For this review, take the finished solid that the model builds, in its own axes (mm). A direction names the side the tool comes from. Round coordinates to 2 decimals unless told otherwise and drop trailing zeros. Write each loop counter-clockwise with the first axis right and the second up, starting at its lowest first coordinate (ties: lowest second). Pieces come first, ordered by that corner, then holes. Notation, with made-up numbers: (63, 22.25) -> (77, 22.25) arc R17 cw to (77, 29.25) -> close; hole circle Ø10 at (83, -32). An arc over 180 degrees is marked (long way). Answer in a Markdown table with one row per item.
from build123d import *

# Parameters (mm, degrees)
SKETCH2_R           = 12.7
BOSS_EXTRUDE1_DEPTH = 38.1
CUT_EXTRUDE1_DEPTH  = 99.465595781


with BuildPart() as part:
    # Sketch2 → Boss-Extrude1 (new body)
    with BuildSketch(Plane.XY):
        with BuildLine():
            Line((-69.85, -36.5125), (69.85, -36.5125))
            Line((69.85, -36.5125), (69.85, -21.43125))
            Line((69.85, -21.43125), (29.639590069, -21.43125))
            ThreePointArc((29.639590069, -21.43125), (0, 36.576), (-29.639590069, -21.43125))
            Line((-29.639590069, -21.43125), (-69.85, -21.43125))
            Line((-69.85, -21.43125), (-69.85, -36.5125))
        make_face()
        with Locations(Location((0, 0, 0), (0, 0, 180))):
            Circle(SKETCH2_R, mode=Mode.SUBTRACT)
    extrude(amount=BOSS_EXTRUDE1_DEPTH)

    # Sketch3 → Cut-Extrude1 (cut, through all)
    with BuildSketch(Plane(origin=(0, -21.43125, 0), x_dir=(1, 0, 0), z_dir=(0, 1, 0))):
        with BuildLine():
            Line((-58.7375, -15.875), (-46.0375, -15.875))
            ThreePointArc((-46.0375, -15.875), (-42.8625, -19.05), (-46.0375, -22.225))
            Line((-46.0375, -22.225), (-58.7375, -22.225))
            ThreePointArc((-58.7375, -22.225), (-61.9125, -19.05), (-58.7375, -15.875))
        make_face()
    cut_extrude1 = extrude(amount=-CUT_EXTRUDE1_DEPTH, mode=Mode.SUBTRACT)

    # Mirror1: Cut-Extrude1 across plane
    add(cut_extrude1.mirror(Plane(origin=(0, 0, 0), x_dir=(0, 0, 1), z_dir=(1, 0, 0))), mode=Mode.SUBTRACT)


solid = part.part
1) For line 1 (Y direction, x = 0, z = 8.5); line 2 (Y direction, x = 57, z = 10.5); line 3 (Y direction, x = -33, z = 13), list the stretches that pass through material, from the lowest coordinate up. Write a range as [from, to].
Solved:
| item | result |
|---|---|
| line 1 | [-36.51, -12.7], [12.7, 36.58] |
| line 2 | [-36.51, -21.43] |
| line 3 | [-36.51, -21.43], [-15.77, 15.77] |
2) Consider section A-A on z = 19.05. State the section outline as (x, y) points.
Solved:
| item | result |
|---|---|
| outline | (-69.85, -36.51) -> (-61.91, -36.51) -> (-61.91, -21.43) -> (-69.85, -21.43) -> close; (-42.86, -36.51) -> (42.86, -36.51) -> (42.86, -21.43) -> (29.64, -21.43) arc R36.58 ccw (long way) to (-29.64, -21.43) -> (-42.86, -21.43) -> close; (61.91, -36.51) -> (69.85, -36.51) -> (69.85, -21.43) -> (61.91, -21.43) -> close; hole circle Ø25.4 at (0, 0) |
3) For faces 1 (the cylindrical face through (-5.86, 11.267, 18.783)), 2 (the cylindrical face through (-61.91, -28.87, 19.12)), list the 3-axis set-ups (+Z, -Z, +X, -X, +Y, -Y) from which the entire face can be reached by the end or side of a thin tool; tool diameter is ignored.
Solved:
| item | result |
|---|---|
| face 1 | +Z, -Z |
| face 2 | +Y, -Y |
4) Consider section D-D on y = 0. State the section outline as (x, z) points.
Solved:
| item | result |
|---|---|
| outline | (-36.58, 0) -> (-12.7, 0) -> (-12.7, 38.1) -> (-36.58, 38.1) -> close; (12.7, 0) -> (36.58, 0) -> (36.58, 38.1) -> (12.7, 38.1) -> close |
5) Consider section B-B on x = -53. State the section outline as (y, z) points (1 decimal).
Solved:
| item | result |
|---|---|
| outline | (-36.5, 0) -> (-21.4, 0) -> (-21.4, 15.9) -> (-36.5, 15.9) -> close; (-36.5, 22.2) -> (-21.4, 22.2) -> (-21.4, 38.1) -> (-36.5, 38.1) -> close |
6) Consider section C-C on y = -31.5. State how many separate pieces and enclosed holes the cut face has, then the cut area to 3 significant figures.
Solved:
| item | result |
|---|---|
| separate pieces | 1 |
| enclosed holes | 2 |
| area | 5,100 mm² |
7) Clearance check with flat-ended pins moving along their axes: pin 1 Ø6.5 at (x, y) = (-54.5, -32) entering from -Z; pin 2 Ø1 at (y, z) = (10.5, 26.5) entering from -X; pin 3 Ø3 at (y, z) = (9.5, 23) entering from -X; pin 4 Ø12 at (y, z) = (4, 26.5) entering from -X. State where each tip first meets the part, or that it passes through.
Solved:
| item | result |
|---|---|
| pin 1 | z = 0 |
| pin 2 | x = -35.18 |
| pin 3 | x = -35.69 |
| pin 4 | x = -36.58 |
8) Mouldability with a two-part tool opening along Y and no side actions: class faces 3 (the flat face through (-1, -36.512, 19)), 4 (the cylindrical face through (61.91, -28.87, 19.12)), 5 (the flat face through (-49, -21.431, 23)) as pulls with the +Y half, pulls with the -Y half, needs draft (parallel to the pull), parting line crosses it, or undercut.
Solved:
| item | result |
|---|---|
| face 3 | pulls with the -Y half |
| face 4 | needs draft |
| face 5 | undercut |
